For this review, take the finished solid that the model builds, in its own axes (mm). Face numbers are marked on the shaded views. A direction names the side the tool comes from. Coordinates: 2 decimals unless noted, no trailing zeros. Order: outer loops, then holes, each group sorted by start corner. A loop starts at its lowest first (then second) coordinate and runs counter-clockwise, first axis right, second up. Notation, with made-up numbers: (-33, 12.5) -> (22, 12.5) arc R14 ccw to (22, 18.5) -> close; hole circle Ø10 at (86.5, 76). An arc over 180 degrees is marked (long way). Return JSON: item names as keys, results as strings. Group by question number.
Item 1: Insertion check: pin 1 (5 mm diameter, centred on x = -2.5, z = 12.5, fed in from +Y); pin 2 (1.5 mm diameter, centred on y = -3.5, z = 2, fed in from -X); pin 3 (3 mm diameter, centred on x = -2.5, z = 7, fed in from -Y). Each pin has a flat end and moves straight along its axis. Give the tip position at first contact, or say it passes through.
Item 2: Take a section at A-A (x = 0). Write out the cut boundary in (y, z), then the cut area to 4 significant figures.
Item 3: Take a section at B-B (y = 0). Write out the cut boundary in (x, z), then the cut area to 3 significant figures.
Item 4: Take a section at D-D (x = -2). Write out the cut boundary in (y, z).
Item 5: Draft analysis for pull direction Y (two halves, no side actions). For the marked faces 4, 5 and 6, state which applies: +Y half, -Y half, draft (parallel to the pull), parting line (faces both ways), or undercut.
Item 6: For line 1 along X through (y, z) = (0, 2.1); line 2 along Z through (x, y) = (-5, -2.5); line 3 along X through (y, z) = (3.75, 2.75), list the stretches that pass through material, from the lowest coordinate up.
Item 7: Take a section at C-C (z = 13.25). Write out the cut boundary in (x, y).
Item 8: Machinability: for the marked faces 1, 2 and 3, which of the approach directions +Z, -Z, +X, -X, +Y, -Y give a long, thin tool a straight path to every point of the face, cutting with its end or side? Answer none if there is none.
```python
from build123d import *

# Parameters (mm, degrees)
SKETCH4_R           = 6.5
BOSS_EXTRUDE1_DEPTH = 6
CUT_EXTRUDE2_DEPTH  = 4
SKETCH7_R           = 2.5
BOSS_EXTRUDE2_DEPTH = 10.33


with BuildPart() as part:
    # Sketch4 → Boss-Extrude1 (new body)
    with BuildSketch(Plane.XY):
        Circle(SKETCH4_R)
    extrude(amount=BOSS_EXTRUDE1_DEPTH)

    # Sketch6 → Cut-Extrude2 (cut)
    with BuildSketch(Plane.XY):
        with BuildLine():
            Line((2.945810333, 2.23879465), (2.718410219, 5.90425659))
            ThreePointArc((2.718410219, 5.90425659), (0, 6.5), (-2.718410219, 5.90425659))
            Line((-2.718410219, 5.90425659), (-2.945810333, 2.23879465))
            ThreePointArc((-2.945810333, 2.23879465), (0, -3.7), (2.945810333, 2.23879465))
        make_face()
    extrude(amount=CUT_EXTRUDE2_DEPTH, mode=Mode.SUBTRACT)

    # Sketch7 → Boss-Extrude2 (add)
    with BuildSketch(Plane.XY.offset(6)):
        Circle(SKETCH7_R)
    extrude(amount=BOSS_EXTRUDE2_DEPTH)


solid = part.part
```
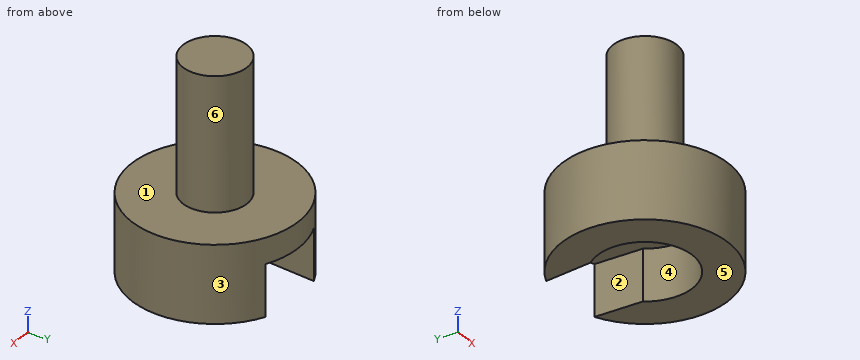
Findings below:
{
 "1": {"pin 1": "stops at y = 2.5", "pin 2": "stops at x = -5.89", "pin 3": "stops at y = -6.35"},
 "2": {"outline": "(-6.5, 0) -> (-3.7, 0) -> (-3.7, 4) -> (6.5, 4) -> (6.5, 6) -> (2.5, 6) -> (2.5, 16.33) -> (-2.5, 16.33) -> (-2.5, 6) -> (-6.5, 6) -> close", "area": "88.85 mm2"},
 "3": {"outline": "(-6.5, 0) -> (-3.7, 0) -> (-3.7, 4) -> (3.7, 4) -> (3.7, 0) -> (6.5, 0) -> (6.5, 6) -> (2.5, 6) -> (2.5, 16.33) -> (-2.5, 16.33) -> (-2.5, 6) -> (-6.5, 6) -> close", "area": "100 mm2"},
 "4": {"outline": "(-6.18, 0) -> (-3.11, 0) -> (-3.11, 4) -> (6.18, 4) -> (6.18, 6) -> (1.5, 6) -> (1.5, 16.33) -> (-1.5, 16.33) -> (-1.5, 6) -> (-6.18, 6) -> close"},
 "5": {"face 4": "undercut", "face 5": "draft", "face 6": "parting line"},
 "6": {"line 1": "x = -6.5 to -3.7, 3.7 to 6.5", "line 2": "z = 0 to 6", "line 3": "x = -5.31 to -2.85, 2.85 to 5.31"},
 "7": {"outline": "circle Ø5 at (0, 0)"},
 "8": {"face 1": "+Z", "face 2": "-Z", "face 3": "+Z, -Z"}
}
